```python
from build123d import *

# Parameters (mm, degrees)
SKETCH_1_R         = 6
EXTRUDE_1_DEPTH    = 5
HOLE_WIZARD_M4_1_D = 3.3


with BuildPart() as part:
    # 草圖1 → 填料-伸長1 (new body)
    with BuildSketch(Plane(origin=(0, 0, 0), x_dir=(1, 0, 0), z_dir=(0, 1, 0))):
        with BuildLine():
            ThreePointArc((-75.637707948, 93.160813309), (-103.923048454, 60), (-118.498484937, 18.923769913))
            ThreePointArc((-118.498484937, 18.923769913), (-108.660524842, -4.035424469), (-83.701905284, -5.024047358))
            ThreePointArc((-83.701905284, -5.024047358), (-32.475952642, -18.75), (-46.201905284, -69.975952642))
            ThreePointArc((-46.201905284, -69.975952642), (-57.825042527, -92.085062668), (-42.860776988, -112.084583222))
            ThreePointArc((-42.860776988, -112.084583222), (0, -120), (42.860776988, -112.084583222))
            ThreePointArc((42.860776988, -112.084583222), (57.825042527, -92.085062668), (46.201905284, -69.975952642))
            ThreePointArc((46.201905284, -69.975952642), (32.475952642, -18.75), (83.701905284, -5.024047358))
            ThreePointArc((83.701905284, -5.024047358), (108.660524842, -4.035424469), (118.498484937, 18.923769913))
            ThreePointArc((118.498484937, 18.923769913), (103.923048454, 60), (75.637707948, 93.160813309))
            ThreePointArc((75.637707948, 93.160813309), (50.835482316, 96.120487137), (37.5, 75))
            ThreePointArc((37.5, 75), (0, 37.5), (-37.5, 75))
            ThreePointArc((-37.5, 75), (-50.835482316, 96.120487137), (-75.637707948, 93.160813309))
        make_face()
        with Locations(Location((0, 0, 0), (0, 0, 270))):
            Circle(SKETCH_1_R, mode=Mode.SUBTRACT)
    extrude(amount=-EXTRUDE_1_DEPTH)

    # M4 螺紋孔1 (through all)
    with Locations(Plane(origin=(0, 0, 0), x_dir=(1, 0, 0), z_dir=(0, 1, 0))):
        with Locations((0, 12), (12, 0), (0, -12), (-12, 0)):
            Hole(HOLE_WIZARD_M4_1_D / 2)


solid = part.part
```
Source: CAD feature listing. Evaluate the final solid. Frame: model axes, mm. Round coordinates to 2 decimals unless told otherwise and drop trailing zeros. Loops run counter-clockwise (first coordinate to the right, second up) from the corner with the lowest first, then second, coordinate; pieces in that order, holes last.
(1) Pull-direction query (X, two-part tool) for faces 1 (the flat face through (-2, -5, 9)), 2 (the cylindrical face through (104.228, -2.465, -59.468)), 3 (the cylindrical face through (108.36, -2.46, 4.24)), 4 (the cylindrical face through (-103.615, -2.465, -60.531)); classes: +X half, -X half, draft (parallel to the pull), parting line (faces both ways), or undercut.
From the geometry:
face 1: draft
face 2: +X half
face 3: undercut
face 4: -X half
(2) Contact query for a flat-ended pin moving along its axis: pin 1 Ø2.5 at (x, z) = (12, 0) entering from +Y. Output: stop coordinate, or through.
From the geometry:
pin 1: passes through
(3) Section query C-C (x = 62). Output: boundary loops of the cut face in (y, z), and give its area (3 significant figures).
From the geometry:
outline: (-5, -98.37) - (0, -98.37) - (0, 0.12) - (-5, 0.12) - close
area: 492 mm2
(4) Section query B-B (z = 37.5). Output: boundary loops of the cut face in (x, y), and give its area (3 significant figures).
From the geometry:
outline: (-27.45, -5) - (27.45, -5) - (27.45, 0) - (-27.45, 0) - close
area: 275 mm2
(5) Material intervals for probe 1 along X at (y, z) = (-3, 12); probe 2 along X at (y, z) = (-3.75, -12); probe 3 along X at (y, z) = (-1.05, -14), sorted ascending.
From the geometry:
probe 1: x = -37.46 to -1.65, 1.65 to 37.46
probe 2: x = -118.57 to -1.65, 1.65 to 118.57
probe 3: x = -118.76 to 118.76
(6) Section query A-A (y = -4.1). Output: boundary loops of the cut face in (x, z), and give its area (3 significant figures).
From the geometry:
outline: (-118.5, -18.92) arc R120 ccw to (-75.64, -93.16) arc R23.39 ccw to (-37.5, -75) arc R37.5 cw to (37.5, -75) arc R23.39 ccw to (75.64, -93.16) arc R120 ccw to (118.5, -18.92) arc R23.39 ccw to (83.7, 5.02) arc R37.5 cw to (46.2, 69.98) arc R23.39 ccw to (42.86, 112.08) arc R120 ccw to (-42.86, 112.08) arc R23.39 ccw to (-46.2, 69.98) arc R37.5 cw to (-83.7, 5.02) arc R23.39 ccw to start; hole circle Ø3.3 at (-12, 0); hole circle Ø12 at (0, 0); hole circle Ø3.3 at (0, -12); hole circle Ø3.3 at (0, 12); hole circle Ø3.3 at (12, 0)
area: 26,400 mm2
